Autodesk Inventor part; units mm, degrees
ref_plane "YZ Plane" through (0, 0, 0) normal (1, 0, 0) x (0, 1, 0)
ref_plane "XZ Plane" through (0, 0, 0) normal (0, 1, 0) x (-1, 0, 0)
ref_plane "XY Plane" through (0, 0, 0) normal (0, 0, 1) x (1, 0, 0)
sketch "Sketch1" plane through (0, 0, 0) normal (1, 0, 0) x (0, 1, 0)
  line L0 (-6.35, -3.6662) -> (-6.35, 3.6662)
  line L1 (-6.35, 3.6662) -> (0, 7.3323)
  line L2 (0, 7.3323) -> (6.35, 3.6662)
  line L3 (6.35, 3.6662) -> (6.35, -3.6662)
  line L4 (6.35, -3.6662) -> (0, -7.3323)
  line L5 (0, -7.3323) -> (-6.35, -3.6662)
  point P0 (0, 0)
  point P1 (0, 0)
  dimension "d0" = 12.7
extrude "Extrusion1" add sketch "Sketch1" along normal blind 193.548
sketch "Sketch2" plane through (0, 0, 0) normal (-1, 0, 0) x (0, 0, 1)
  point P0 (0, 0)
  point P1 (0, 0)
hole "Hole1" at (0, 0, 0) direction (1, 0, 0) diameter 3.9624 end through all
properties part number "STOCK,SHAFT,HEX,HOOD,WHEELS" material "Aluminum 6061"
For this review, take the finished solid that the model builds, in its own axes (mm). Round coordinates to 2 decimals unless told otherwise and drop trailing zeros. Write each loop counter-clockwise with the first axis right and the second up, starting at its lowest first coordinate (ties: lowest second). Pieces come first, ordered by that corner, then holes. Notation, with made-up numbers: (39, 78.25) -> (94, 78.25) arc R22 cw to (94, 113.25) -> close; hole circle Ø1 at (81, 22). An arc over 180 degrees is marked (long way). Use one line per item in the form item = value.
Q1. Consider section B-B (x = 169). State the section outline as (y, z) points.
Resolved:
outline = (-6.35, -3.67) -> (0, -7.33) -> (6.35, -3.67) -> (6.35, 3.67) -> (0, 7.33) -> (-6.35, 3.67) -> close; hole circle Ø3.96 at (0, 0)
Q2. Consider section D-D (y = 3.75). State the section outline as (x, z) points.
Resolved:
outline = (0, -5.17) -> (193.55, -5.17) -> (193.55, 5.17) -> (0, 5.17) -> close
Q3. Consider section A-A (z = 0). State the section outline as (x, y) points.
Resolved:
outline = (0, -6.35) -> (193.55, -6.35) -> (193.55, -1.98) -> (0, -1.98) -> close; (0, 1.98) -> (193.55, 1.98) -> (193.55, 6.35) -> (0, 6.35) -> close
Q4. To check wall thickness, follow probe 1 along Y at (x, z) = (116.5, 0); probe 2 along Z at (x, y) = (116, 0); probe 3 along Z at (x, y) = (62, 0.25). State the ranges of each line that lie inside material, in increasing order. Write a range as from..to.
Resolved:
probe_1 = -6.35..-1.98, 1.98..6.35
probe_2 = -7.33..-1.98, 1.98..7.33
probe_3 = -7.19..-1.97, 1.97..7.19
Q5. Clearance check with flat-ended pins moving along their axes: pin 1 Ø6 at (y, z) = (0, 5) entering from -X; pin 2 Ø6 at (x, y) = (84.5, 1) entering from +Z; pin 3 Ø6 at (x, y) = (79, -0.5) entering from -Z. State where each tip first meets the part, or that it passes through.
Resolved:
pin_1 = 0
pin_2 = 7.33
pin_3 = -7.33
Q6. Consider section C-C (y = -4.75). State the section outline as (x, z) points, then the cut area to 3 significant figures.
Resolved:
outline = (0, -4.59) -> (193.55, -4.59) -> (193.55, 4.59) -> (0, 4.59) -> close
area = 1,780 mm²
